```python
from build123d import *

# Parameters (mm, degrees)
SKETCH1_R           = 80
BOSS_EXTRUDE1_DEPTH = 19.2


with BuildPart() as part:
    # Sketch1 → Boss-Extrude1 (new body)
    with BuildSketch(Plane(origin=(0, 0, 0), x_dir=(1, 0, 0), z_dir=(0, 1, 0))):
        with Locations(Location((0, 0, 0), (0, 0, 270))):
            Circle(SKETCH1_R)
        with BuildLine():
            ThreePointArc((1.638299788, 70.98109589), (0, 75.6), (-1.638299788, 70.98109589))
            ThreePointArc((-1.638299788, 70.98109589), (-50.204581464, 50.204581464), (-70.98109589, 1.638299788))
            ThreePointArc((-70.98109589, 1.638299788), (-75.6, 0), (-70.98109589, -1.638299788))
            ThreePointArc((-70.98109589, -1.638299788), (-50.204581464, -50.204581464), (-1.638299788, -70.98109589))
            ThreePointArc((-1.638299788, -70.98109589), (0, -75.6), (1.638299788, -70.98109589))
            ThreePointArc((1.638299788, -70.98109589), (50.204581464, -50.204581464), (70.98109589, -1.638299788))
            ThreePointArc((70.98109589, -1.638299788), (75.6, 0), (70.98109589, 1.638299788))
            ThreePointArc((70.98109589, 1.638299788), (50.204581464, 50.204581464), (1.638299788, 70.98109589))
        make_face(mode=Mode.SUBTRACT)
    extrude(amount=BOSS_EXTRUDE1_DEPTH)


solid = part.part
```
Source: CAD feature listing. Evaluate the final solid. Frame: model axes, mm. A direction names the side the tool comes from. Round coordinates to 2 decimals unless told otherwise and drop trailing zeros. Loops run counter-clockwise (first coordinate to the right, second up) from the corner with the lowest first, then second, coordinate; pieces in that order, holes last. Notation, with made-up numbers: M 57.5,64.5 L 106.5,64.5 A15 ccw 106.5,68.5 Z; hole C 63.25,-0.5 d11. An arc over 180 degrees is marked long. Use a Markdown table: item, result. Add a question column.
1. Section query A-A on y = 8.5. Return the cut outline in (x, z).
2. Contact query for flat-ended pins moving along their axis: P1, Ø3, axis at x = 33.5, y = 16, coming from the +Z side; P2, Ø2, axis at x = -9, y = 11, coming from the -Z side; P3, Ø3, axis at x = 73, z = 0, coming from the -Y side; P4, Ø10, axis at x = 29, y = 17, coming from the -Z side. Output: stop coordinate, or through.
3. Line query: line 1 (X direction, y = 6.5, z = -42); line 2 (X direction, y = 13.5, z = 73); line 3 (Z direction, x = 4, y = 10.5). Output: solid intervals per line, ascending.
4. Reachability of faces 5 (the cylindrical face through (49.666, 9.466, 50.738)), 6 (the flat face through (71, 0, -6)) from +Z, -Z, +X, -X, +Y, -Y: full face, straight path, thin tool, end or side. Return the list, or none.
5. Section query C-C on x = -73. Return the cut outline in (y, z).
6. Section query B-B on z = -28. Return the cut outline in (x, y), then the cut area to 3 significant figures.
7. Mould query, pull axis Z, two halves, no side actions, for faces 1 (the cylindrical face through (-49.666, 9.466, -50.738)), 2 (the cylindrical face through (-78.1, 9.47, -17.34)), 3 (the flat face through (71, 19.2, -6)), 4 (the cylindrical face through (75.6, 9.5, 0.1)). Classes: pulls with the +Z half, pulls with the -Z half, needs draft (parallel to the pull), parting line crosses it, or undercut.
Reported:
| question | item | result |
|---|---|---|
| 1 | outline | C 0,0 d160; hole M -70.98,-1.64 A71 ccw -1.64,-70.98 A2.6 ccw long 1.64,-70.98 A71 ccw 70.98,-1.64 A2.6 ccw long 70.98,1.64 A71 ccw 1.64,70.98 A2.6 ccw long -1.64,70.98 A71 ccw -70.98,1.64 A2.6 ccw long Z |
| 2 | P1 | stops at z = 73.32 |
| 2 | P2 | stops at z = -79.6 |
| 2 | P3 | passes through |
| 2 | P4 | stops at z = -76.32 |
| 3 | line 1 | x = -68.09 to -57.25, 57.25 to 68.09 |
| 3 | line 2 | x = -32.73 to -2.6, 2.6 to 32.73 |
| 3 | line 3 | z = -79.9 to -70.89, 70.89 to 79.9 |
| 4 | face 5 | +Y, -Y |
| 4 | face 6 | +Z, -Z, +X, -X, -Y |
| 5 | outline | M 0,-32.73 L 19.2,-32.73 L 19.2,-2.6 L 0,-2.6 Z; M 0,2.6 L 19.2,2.6 L 19.2,32.73 L 0,32.73 Z |
| 6 | outline | M -74.94,0 L -65.25,0 L -65.25,19.2 L -74.94,19.2 Z; M 65.25,0 L 74.94,0 L 74.94,19.2 L 65.25,19.2 Z |
| 6 | area | 372 mm² |
| 7 | face 1 | undercut |
| 7 | face 2 | parting line crosses it |
| 7 | face 3 | needs draft |
| 7 | face 4 | undercut |
